Autodesk Fusion 360 part; units mm, degrees
sketch "スケッチ1" plane through (0, 0, 0) normal (0, 0, 1) x (1, 0, 0)
  line L0 (-15.5, 115) -> (-74.5, 115)
  line L1 (-74.5, 115) -> (-74.5, -115)
  line L2 (-74.5, -115) -> (-15.5, -115)
  line L3 (74.5, -25) -> (74.5, 105)
  line L4 (68.0217, 105) -> (-74.5, -115) construction
  line L5 (-74.5, 115) -> (39.1174, -60.3826) construction
  line L6 (-15.5, 115) -> (-15.5, 105)
  line L7 (-15.5, 105) -> (74.5, 105)
  line L8 (-74.5, -115) -> (-15.5, -115) construction
  line L9 (74.5, -25) -> (-15.5, -115)
  dimension "d2" = 230
  dimension "d5" = 59
extrude "押し出し1" add sketch "スケッチ1" along normal blind 6
chamfer "面取り1" distance 20 angle 45 2 edges at (-74.5, -115, 3) (-74.5, 115, 3)
sketch "スケッチ2" plane through (0, 0, 6) normal (0, 0, 1) x (-1, 0, 0)
  line L0 (54.5, -115) -> (74.5, -95)
  line L1 (74.5, -95) -> (74.5, 95)
  line L2 (74.5, 95) -> (54.5, 115)
  line L3 (54.5, 115) -> (15.5, 115)
  line L4 (15.5, 115) -> (-74.5, 25)
  line L5 (-74.5, 25) -> (-74.5, -105)
  line L6 (-74.5, -105) -> (15.5, -105)
  line L7 (15.5, -105) -> (15.5, -115)
  line L8 (15.5, -115) -> (54.5, -115)
  line L9 (-74.5, -105) -> (-34.5, -105) construction
  line L10 (-34.5, -105) -> (-34.5, -75) construction
  line L11 (-34.5, -75) -> (-74.5, -75) construction
  line L12 (-74.5, -75) -> (-74.5, -105) construction
  line L13 (-34.5, -75) -> (-34.5, -25) construction
  point P0 (-34.5, -75)
  point P1 (-34.5, -25)
  dimension "d10" = 40
  dimension "d11" = 30
  dimension "d12" = 50
hole "穴1" at (34.5, 75, 6) at (34.5, 25, 6) direction (0, 0, -1) diameter 18 end through all
equation "d5 = 20 mm + 39 mm"
Build history of the part. All positions in model axes, mm. A direction names the side the tool comes from. Coordinates: 2 decimals unless noted, no trailing zeros. Order: outer loops, then holes, each group sorted by start corner. A loop starts at its lowest first (then second) coordinate and runs counter-clockwise, first axis right, second up.
Item 1: Saw through at B-B on x = 34.5. List the corners of the cut face in (y, z), then the cut area to 3 significant figures.
Filled in:
outline: (-65, 0) - (16, 0) - (16, 6) - (-65, 6) - close; (34, 0) - (66, 0) - (66, 6) - (34, 6) - close; (84, 0) - (105, 0) - (105, 6) - (84, 6) - close
area: 804 mm2
Item 2: Drill centre lines: L1, parallel to X at y = 75, z = 3.75; L2, parallel to Y at x = 34.5, z = 1.3; L3, parallel to X at y = 71, z = 4.2. Where is each one in solid material? Low to high.
Filled in:
L1: x = -74.5 to 25.5, 43.5 to 74.5
L2: y = -65 to 16, 34 to 66, 84 to 105
L3: x = -74.5 to 26.44, 42.56 to 74.5
Item 3: Saw through at A-A on y = 75. List the corners of the cut face in (x, z).
Filled in:
outline: (-74.5, 0) - (25.5, 0) - (25.5, 6) - (-74.5, 6) - close; (43.5, 0) - (74.5, 0) - (74.5, 6) - (43.5, 6) - close
Item 4: Mould opens along Y. For faces 1 (the cylindrical face through (26.91, 70.16, 2.96)), 2 (the flat face through (74.5, 39, 3)), 3 (the flat face through (-35, -115, 3)) say: released by +Y, released by -Y, zero draft, split by the parting line, or undercut.
Filled in:
face 1: undercut
face 2: zero draft
face 3: released by -Y
Item 5: Saw through at C-C on z = 3. List the corners of the cut face in (x, y), then the cut area to 3 significant figures.
Filled in:
outline: (-74.5, -95) - (-54.5, -115) - (-15.5, -115) - (74.5, -25) - (74.5, 105) - (-15.5, 105) - (-15.5, 115) - (-54.5, 115) - (-74.5, 95) - close; hole circle Ø18 at (34.5, 25); hole circle Ø18 at (34.5, 75)
area: 28,400 mm2
Item 6: Tool access for faces 4 (the flat face through (-64.6, -104.9, 3)), 5 (the flat face through (-15.5, 110, 3)): list every direction of +Z, -Z, +X, -X, +Y, -Y with a clear straight run to the whole face (end or side of a thin tool).
Filled in:
face 4: +Z, -Z, -X, -Y
face 5: +Z, -Z, +X, +Y
Item 7: Saw through at D-D on y = 25.5. List the corners of the cut face in (x, z), then the cut area to 3 significant figures.
Filled in:
outline: (-74.5, 0) - (25.51, 0) - (25.51, 6) - (-74.5, 6) - close; (43.49, 0) - (74.5, 0) - (74.5, 6) - (43.49, 6) - close
area: 786 mm2
Item 8: Drop flat-ended pins along their axis: pin 1 Ø3 at (x, z) = (49, 2) entering from +Y; pin 2 Ø3 at (y, z) = (-52.5, 5.5) entering from +X; pin 3 Ø12 at (x, y) = (-54, -74.5) entering from -Z; pin 4 Ø3 at (y, z) = (112, 2.5) entering from +X. Give the stop position or say it passes through.
Filled in:
pin 1: stops at y = 105
pin 2: stops at x = 48.5
pin 3: stops at z = 0
pin 4: stops at x = -15.5
